Model file for the job. Use its own axes, mm. Face numbers are marked on the shaded views. A direction names the side the tool comes from. Round coordinates to 2 decimals unless told otherwise and drop trailing zeros. Loops run counter-clockwise (first coordinate to the right, second up) from the corner with the lowest first, then second, coordinate; pieces in that order, holes last. Notation, with made-up numbers: (64, 44.5) - (92, 44.5) arc R6 cw to (92, 53.5) - close; hole circle Ø3 at (-20, 34). An arc over 180 degrees is marked (long way). Answer as a JSON object with one key per item and string values.
from build123d import *

# Parameters (mm, degrees)
BOX_W        = 10
BOX_H        = 10
BOX_DEPTH    = 30
BOX001_W     = 10
BOX001_H     = 10
BOX001_DEPTH = 20
BOX002_W     = 10
BOX002_H     = 10
BOX002_DEPTH = 20
BOX003_W     = 10
BOX003_H     = 10
BOX003_DEPTH = 10
BOX004_W     = 10
BOX004_H     = 10
BOX004_DEPTH = 10
BOX005_W     = 10
BOX005_H     = 10
BOX005_DEPTH = 10


with BuildPart() as cube:
    # Box → Box (new body)
    with BuildSketch(Plane.XY):
        with Locations((5, 5)):
            Rectangle(BOX_W, BOX_H)
    extrude(amount=BOX_DEPTH)


with BuildPart() as cube001:
    # Box001 → Box001 (new body)
    with BuildSketch(Plane(origin=(10, 0, 0), x_dir=(1, 0, 0), z_dir=(0, 0, 1))):
        with Locations((5, 5)):
            Rectangle(BOX001_W, BOX001_H)
    extrude(amount=BOX001_DEPTH)


with BuildPart() as cube002:
    # Box002 → Box002 (new body)
    with BuildSketch(Plane(origin=(0, 10, 0), x_dir=(1, 0, 0), z_dir=(0, 0, 1))):
        with Locations((5, 5)):
            Rectangle(BOX002_W, BOX002_H)
    extrude(amount=BOX002_DEPTH)


with BuildPart() as cube003:
    # Box003 → Box003 (new body)
    with BuildSketch(Plane(origin=(20, 0, 0), x_dir=(1, 0, 0), z_dir=(0, 0, 1))):
        with Locations((5, 5)):
            Rectangle(BOX003_W, BOX003_H)
    extrude(amount=BOX003_DEPTH)


with BuildPart() as cube004:
    # Box004 → Box004 (new body)
    with BuildSketch(Plane(origin=(0, 20, 0), x_dir=(1, 0, 0), z_dir=(0, 0, 1))):
        with Locations((5, 5)):
            Rectangle(BOX004_W, BOX004_H)
    extrude(amount=BOX004_DEPTH)


with BuildPart() as fusion:
    # Box005 → Box005 (new body)
    with BuildSketch(Plane(origin=(10, 10, 0), x_dir=(1, 0, 0), z_dir=(0, 0, 1))):
        with Locations((5, 5)):
            Rectangle(BOX005_W, BOX005_H)
    extrude(amount=BOX005_DEPTH)

    # Fusion: union Cube, Cube001, Cube002, Cube003, Cube004
    add(cube.part)
    add(cube001.part)
    add(cube002.part)
    add(cube003.part)
    add(cube004.part)


solid = fusion.part
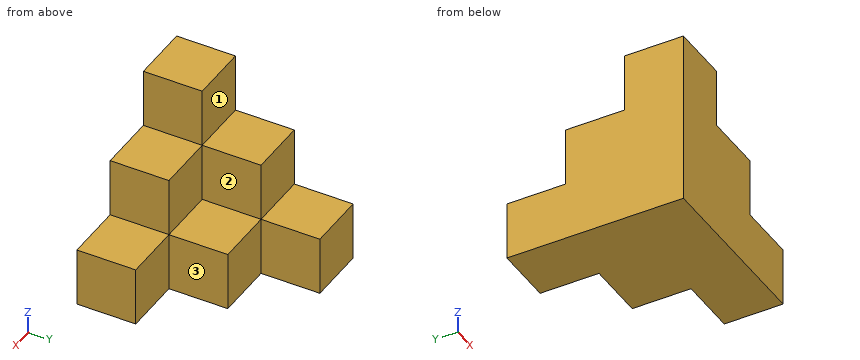
1) Slice it at C-C on z = 13.75. List the corners of the cut face in (x, y).
Values follow:
{"outline": "(0, 0) - (20, 0) - (20, 10) - (10, 10) - (10, 20) - (0, 20) - close"}
2) Drop flat-ended pins along their axis: P1, Ø4, axis at y = 23.5, z = 14.5, coming from the -X side; P2, Ø11, axis at y = 24, z = 5.5, coming from the +X side; P3, Ø3, axis at x = 16.5, z = 6, coming from the +Y side; P4, Ø4, axis at x = 11, y = 26.5, coming from the +Z side. Give the stop position or say it passes through.
Values follow:
{"P1": "through", "P2": "x = 20", "P3": "y = 20", "P4": "z = 10"}
3) Tool access for the marked faces 1, 2 and 3: list every direction of +Z, -Z, +X, -X, +Y, -Y with a clear straight run to the whole face (end or side of a thin tool).
Values follow:
{"face 1": "+Z, +X, -X, +Y", "face 2": "+Z, +X, +Y", "face 3": "+Z, -Z, +X, +Y"}
4) Probe probe 1 along Z at (x, y) = (7.75, 18); probe 2 along X at (y, z) = (1.5, 28.5). List the from-to ranges inside material, lowest first.
Values follow:
{"probe 1": "0 to 20", "probe 2": "0 to 10"}
5) Slice it at A-A on y = 6.75. List the corners of the cut face in (x, z).
Values follow:
{"outline": "(0, 0) - (30, 0) - (30, 10) - (20, 10) - (20, 20) - (10, 20) - (10, 30) - (0, 30) - close"}
